Can you work these out from the model? Positions are in its coordinate system, mm. A direction names the side the tool comes from. Give positions to 0.01 mm unless a question says otherwise; leave off trailing zeros. Order: outer loops, then holes, each group sorted by start corner. A loop starts at its lowest first (then second) coordinate and runs counter-clockwise, first axis right, second up. Notation, with made-up numbers: (-10.75, 82) - (22.25, 82) arc R36 cw to (22.25, 118) - close; hole circle Ø6 at (-5.75, 20.25). An arc over 180 degrees is marked (long way). Return JSON: item names as keys, results as strings.
```python
from build123d import *
from OCP.BRepFilletAPI import BRepFilletAPI_MakeChamfer

# Parameters (mm, degrees)
EXTRUDE_THIN1_DEPTH = 7.5438
SKETCH4_R           = 2.0828
CUT_EXTRUDE1_DEPTH  = 72.173542096
SKETCH5_R           = 2.0828
CUT_EXTRUDE2_DEPTH  = 72.173542096
CHAMFER1_SIZE       = 1.324792988
CHAMFER1_SIZE_2     = 1.524
CIRPATTERN1_COUNT   = 2
CIRPATTERN1_ANGLE   = 90


with BuildPart() as part:
    # Sketch1 → Extrude-Thin1 (new, symmetric)
    with BuildSketch(Plane.XY):
        with BuildLine():
            Line((-50.8, 50.8), (-50.8, 3.048))
            ThreePointArc((-50.8, 3.048), (-49.907261469, 0.892738531), (-47.752, 0))
            Line((-47.752, 0), (0, 0))
            Line((0, 0), (0, 1.524))
            Line((0, 1.524), (-47.752, 1.524))
            ThreePointArc((-47.752, 1.524), (-48.829630735, 1.970369265), (-49.276, 3.048))
            Line((-49.276, 3.048), (-49.276, 50.8))
            Line((-49.276, 50.8), (-50.8, 50.8))
        make_face()
    extrude(amount=EXTRUDE_THIN1_DEPTH, both=True)

    # Sketch4 → Cut-Extrude1 (cut, through all)
    with BuildSketch(Plane(origin=(0, 1.524, 0), x_dir=(1, 0, 0), z_dir=(0, 1, 0))):
        with Locations(Location((-7.5438, 0, 0), (0, 0, 270))):
            Circle(SKETCH4_R)
        with Locations(Location((-38.0238, 0, 0), (0, 0, 270))):
            Circle(SKETCH4_R)
    extrude(amount=-CUT_EXTRUDE1_DEPTH, mode=Mode.SUBTRACT)

    # Sketch5 → Cut-Extrude2 (cut, through all)
    with BuildSketch(Plane(origin=(-49.276, 0, 0), x_dir=(0, 0, -1), z_dir=(1, 0, 0))):
        with Locations(Location((0, 43.18, 0), (0, 0, 90))):
            Circle(SKETCH5_R)
        with Locations(Location((0, 17.78, 0), (0, 0, 90))):
            Circle(SKETCH5_R)
    extrude(amount=-CUT_EXTRUDE2_DEPTH, mode=Mode.SUBTRACT)

    # Chamfer1
    chamfer1_edges_1 = [part.edges().sort_by_distance(p)[0] for p in [
        (-7.5438, 1.524, -2.0828),
    ]]
    chamfer1_side_1 = [part.faces().sort_by_distance(p)[0] for p in [
        (-7.5438, 1.524, -2.10929586),
    ]]
    chamfer1_edges_2 = [part.edges().sort_by_distance(p)[0] for p in [
        (-38.0238, 1.524, -2.0828),
    ]]
    chamfer1_side_2 = [part.faces().sort_by_distance(p)[0] for p in [
        (-38.0238, 1.524, -2.10929586),
    ]]
    chamfer1_edges_3 = [part.edges().sort_by_distance(p)[0] for p in [
        (-49.276, 41.0972, 0),
    ]]
    chamfer1_side_3 = [part.faces().sort_by_distance(p)[0] for p in [
        (-49.276, 41.07070414, 0),
    ]]
    chamfer1_edges_4 = [part.edges().sort_by_distance(p)[0] for p in [
        (-49.276, 15.6972, 0),
    ]]
    chamfer1_side_4 = [part.faces().sort_by_distance(p)[0] for p in [
        (-49.276, 15.67070414, 0),
    ]]
    chamfer1 = BRepFilletAPI_MakeChamfer(part.part.solid().wrapped)
    for e in chamfer1_edges_1:
        chamfer1.Add(CHAMFER1_SIZE - 0.0001, CHAMFER1_SIZE_2 - 0.0001, e.wrapped, chamfer1_side_1[0].wrapped)
    for e in chamfer1_edges_2:
        chamfer1.Add(CHAMFER1_SIZE - 0.0001, CHAMFER1_SIZE_2 - 0.0001, e.wrapped, chamfer1_side_2[0].wrapped)
    for e in chamfer1_edges_3:
        chamfer1.Add(CHAMFER1_SIZE - 0.0001, CHAMFER1_SIZE_2 - 0.0001, e.wrapped, chamfer1_side_3[0].wrapped)
    for e in chamfer1_edges_4:
        chamfer1.Add(CHAMFER1_SIZE - 0.0001, CHAMFER1_SIZE_2 - 0.0001, e.wrapped, chamfer1_side_4[0].wrapped)
    add(Compound.cast(chamfer1.Shape()), mode=Mode.REPLACE)  # a hair under: the kernel refuses the full size


with BuildPart() as cirpattern1_1:
    # CirPattern1: pattern copy
    add(part.part.rotate(Axis((-7.5438, 0, 0), (0, -1, 0)), 1 * CIRPATTERN1_ANGLE / (CIRPATTERN1_COUNT - 1)))

    # Combine1: union part
    add(part.part)


solid = cirpattern1_1.part
```
1. If I drill on L1, parallel to Z at x = -5, y = 4; L2, parallel to Y at x = -13, z = -11.5; L3, parallel to X at y = 43, z = -43, over which ranges is the centre line in solid material (lowest first)? Write a range as [from, to].
Checks:
{"L1": "[-43.26, -41.73]", "L2": "[0, 1.52]", "L3": "[-15.09, -9.84], [-5.25, 0]"}
2. On a 3-axis mill with a long thin cutter (end or side, diameter ignored), from which of +Z, -Z, +X, -X, +Y, -Y can I reach the whole of each face in a straight line? I mean faces 1 (the face through (-8, 27, -41.732)), 2 (the face through (-50, 14, -7.544)), 3 (the face through (-49.276, 27, 0)). Say none if no direction works.
Checks:
{"face 1": "+Z, +X, -X, +Y", "face 2": "-Z, -X, +Y, -Y", "face 3": "+Z, -Z, +X, +Y"}
3. Suppose I cut it at A-A (y = 32). List the corners of the cut face in (x, z) for me.
Checks:
{"outline": "(-50.8, -7.54) - (-49.28, -7.54) - (-49.28, 7.54) - (-50.8, 7.54) - close; (-15.09, -43.26) - (0, -43.26) - (0, -41.73) - (-15.09, -41.73) - close"}
4. For pin 1 Ø12 at (y, z) = (22, 0.5) entering from +X; pin 2 Ø2.5 at (x, z) = (-7.54, 0) entering from -Y; pin 3 Ø16.5 at (x, y) = (-4.5, 35) entering from +Z; pin 4 Ø12 at (x, z) = (-6, -23) entering from +Y, each with a flat end and sliding along its axis, tell me the tip position at first contact or that it passes through.
Checks:
{"pin 1": "x = -49.28", "pin 2": "through", "pin 3": "z = -41.73", "pin 4": "y = 1.52"}
5. Suppose I cut it at C-C (y = 43.18). State how many separate pieces and enclosed holes the cut face has, plus the area to 3 significant figures.
Checks:
{"separate pieces": "4", "enclosed holes": "0", "area": "29.3 mm^2"}
